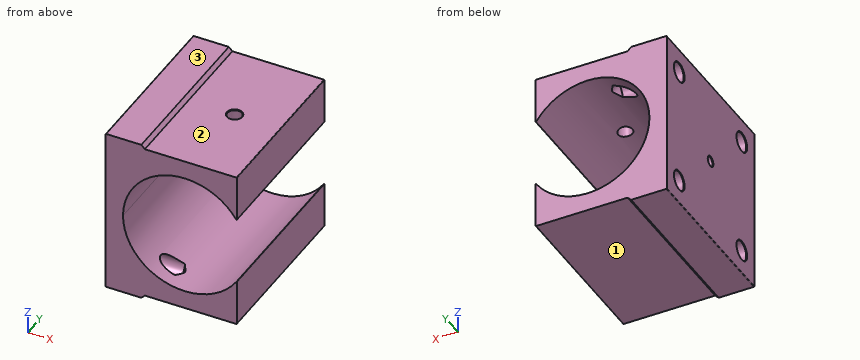
Autodesk Inventor part; units mm, degrees
ref_plane "YZ Plane" through (0, 0, 0) normal (1, 0, 0) x (0, 1, 0)
ref_plane "XZ Plane" through (0, 0, 0) normal (0, 1, 0) x (-1, 0, 0)
ref_plane "XY Plane" through (0, 0, 0) normal (0, 0, 1) x (1, 0, 0)
sketch "Boceto1" plane through (0, 0, 0) normal (0, 1, 0) x (-1, 0, 0)
  line L0 (10.2901, 15.6998) -> (10.2901, -54.8002)
  line L1 (10.2901, -54.8002) -> (-6.2099, -54.8002)
  line L2 (-44.9099, -53.3002) -> (-44.9099, 14.1998)
  line L3 (-6.2099, 15.6998) -> (10.2901, 15.6998)
  line L4 (10.2901, 15.6998) -> (-6.2099, 15.6998)
  line L5 (-6.2099, 15.6998) -> (-6.2099, 14.1998)
  line L6 (-6.2099, 14.1998) -> (-44.9099, 14.1998)
  line L7 (10.2901, -54.8002) -> (-6.2099, -54.8002)
  line L8 (-6.2099, -54.8002) -> (-6.2099, -53.3002)
  line L9 (-6.2099, -53.3002) -> (-44.9099, -53.3002)
  circle A0 centre (-23.0099, -19.5502) radius 26
  point P0 (0, 0)
  point P1 (-44.9099, -5.5363)
  point P2 (-44.9099, -33.5641)
  dimension "d0" = 70.5
  dimension "d3" = 16.5
  dimension "d4" = 1.5
  dimension "d5" = 1.5
  dimension "d6" = 55.2
  dimension "d7" = 67.5
  dimension "d8" = 52
  dimension "d9" = 33.3
  dimension "d10" = 33.75
extrude "Extrusión1" add sketch "Boceto1" along normal blind 70 contours L0 L1 L8 L9 L2 A0 L6 L5 L3
fillet "Empalme1" radius 0.25 2 edges at (-10.2901, 35, 15.6998) (-10.2901, 35, -54.8002)
chamfer "Chaflán1" distance 1.5 angle 45 1 edges at (6.2099, 35, 15.6998)
chamfer "Chaflán2" distance 1.5 angle 45 1 edges at (6.2099, 35, -54.8002)
sketch "Boceto2" plane through (-10.2901, 0, -54.5502) normal (-1, 0, 0) x (0, 0, 1)
  line L0 (9, 70) -> (61, 70)
  line L1 (35, 70) -> (35, 0)
  line L2 (0, 0) -> (70, 0)
  line L3 (35, 35) -> (-0.338, 35)
  line L4 (-0.338, 35) -> (70.438, 35)
  line L5 (35, 35) -> (59.975, 35)
  line L6 (35, 35) -> (10, 35)
  line L7 (10, 35) -> (10, 60)
  line L8 (10, 60) -> (60, 60)
  line L9 (60, 60) -> (60, 10)
  line L10 (60, 10) -> (10, 10)
  line L11 (10, 10) -> (10, 60)
  circle A0 centre (10, 60) radius 4
  circle A1 centre (60, 60) radius 4
  circle A2 centre (10, 10) radius 4
  circle A3 centre (60, 10) radius 4
  circle A4 centre (35, 35) radius 2
  point P0 (54.5502, 0)
  point P1 (49.0139, 70)
  point P2 (20.9861, 70)
  dimension "d23" = 25
  dimension "d24" = 50
  dimension "d25" = 50
  dimension "d26" = 8
  dimension "d27" = 8
  dimension "d28" = 8
  dimension "d29" = 8
  dimension "d30" = 4
  dimension "d73" = 25
hole "Agujero1" at (-10.2901, 60, -44.5502) at (-10.2901, 60, 5.4498) at (-10.2901, 10, -44.5502) at (-10.2901, 10, 5.4498) direction (1, 0, 0) diameter 8 depth 26 tip angle 118
thread "Rosca1"
thread "Rosca2"
thread "Rosca3"
thread "Rosca4"
hole "Agujero2" at (-10.2901, 35, -19.5502) direction (1, 0, 0) diameter 4 depth 26 tip angle 118
thread "Rosca5"
chamfer "Chaflán3" distance 0.25 angle 45 5 edges at (-10.2901, 60, -48.5502) (-10.2901, 60, 1.4498) (-10.2901, 10, -48.5502) (-10.2901, 10, 1.4498) (-10.2901, 35, -21.5502)
sketch "Boceto3" plane through (44.9099, 0, 14.1998) normal (0, 0, 1) x (1, 0, 0)
  point P0 (-44.9099, 0)
sketch "Boceto4" plane through (44.9099, 0, 14.1998) normal (0, 0, 1) x (1, 0, 0)
  line L0 (-38.7, 0) -> (-38.7, 70)
  line L1 (-38.7, 0) -> (-38.7, 70)
  line L2 (-47.9, 70) -> (0, 70)
  line L3 (-38.7, 70) -> (0, 70)
  line L4 (0, 0) -> (0, 70)
  line L5 (0, 70) -> (0, 0)
  line L6 (0, 0) -> (-38.7, 0)
  line L7 (-47.9, 0) -> (0, 0)
  line L8 (-19.35, 0) -> (-19.35, 70)
  line L9 (-19.35, 35) -> (-14.4981, 35)
  line L10 (-14.4981, 35) -> (-25.37, 35)
  circle A0 centre (-19.35, 35) radius 3
  point P0 (-44.9099, 0)
  dimension "d58" = 6
hole "Agujero3" at (25.5599, 35, 14.1998) direction (0, 0, -1) diameter 6 depth 26 tip angle 118
thread "Rosca6"
chamfer "Chaflán4" distance 0.25 angle 45 1 edges at (25.5599, 38, 14.1998)
fillet "Empalme2" radius 0.1 2 edges at (44.9099, 35, -5.5363) (44.9099, 35, -33.5641)
fillet "Empalme3" radius 0.2 2 edges at (44.9099, 35, -53.3002) (44.9099, 35, 14.1998)
properties part number "Soporte de Motor" material "Aluminio 6061"
Here's how the part is built. I have some questions about the finished solid (model axes, mm). Face numbers are marked on the shaded views. A direction names the side the tool comes from. Coordinates: 2 decimals unless noted, no trailing zeros. Write each loop counter-clockwise with the first axis right and the second up, starting at its lowest first coordinate (ties: lowest second). Pieces come first, ordered by that corner, then holes.
Item 1: Will these pins go through, and if not, where does the flat tip stop? pin 1 (6.5 mm diameter, centred on y = 60, z = 5.45, fed in from -X); pin 2 (5 mm diameter, centred on y = 10, z = -44.55, fed in from -X); pin 3 (10 mm diameter, centred on x = 34.5, y = 43, fed in from +Z); pin 4 (3.5 mm diameter, centred on y = 35, z = -19.55, fed in from +X).
Item 2: I want a section at D-D on z = -3. Write out the boundary of the cut face in (x, y).
Item 3: I want a section at B-B on x = -5. Write out the boundary of the cut face in (y, z), and give its area (3 significant figures).
Item 4: If I drill on line 1 (Z direction, x = -5.5, y = 35); line 2 (X direction, y = 35, z = 10.75); line 3 (Y direction, x = 1.5, z = 3), over which ranges is the centre line in solid material (lowest first)?
Item 5: On a 3-axis mill with a long thin cutter (end or side, diameter ignored), from which of +Z, -Z, +X, -X, +Y, -Y can I reach the whole of each face in a straight line? I mean the marked faces 1, 2 and 3. Say none if no direction works.
Item 6: I want a section at A-A on y = 60. Count the separate pieces of the cut face and the enclosed holes in it, and give its area (3 significant figures).
Item 7: I want a section at C-C on x = 35. Write out the boundary of the cut face in (y, z), and give its area (3 significant figures).
Findings below:
1. pin 1: stops at x = 16.16
1. pin 2: stops at x = 16.61
1. pin 3: stops at z = 14.2
1. pin 4: passes through
2. outline: (-10.29, 0) - (2.96, 0) - (2.96, 70) - (-10.29, 70) - close; (43.06, 0) - (44.91, 0) - (44.91, 70) - (43.06, 70) - close
3. outline: (0, -54.8) - (70, -54.8) - (70, 15.7) - (0, 15.7) - close; hole circle Ø8 at (10, -44.55); hole circle Ø8 at (10, 5.45); hole circle Ø4 at (35, -19.55); hole circle Ø8 at (60, -44.55); hole circle Ø8 at (60, 5.45)
3. area: 4,720 mm2
4. line 1: z = -54.8 to -21.55, -17.55 to 15.7
4. line 2: x = -10.29 to 22.56, 28.56 to 44.91
4. line 3: y = 0 to 6.84, 13.16 to 56.84, 63.16 to 70
5. face 1: -Z, +X, +Y, -Y
5. face 2: +Z, +X, +Y, -Y
5. face 3: +Z, +X, -X, +Y, -Y
6. separate pieces: 3
6. enclosed holes: 0
6. area: 1,340 mm2
7. outline: (0, -53.3) - (70, -53.3) - (70, -42.62) - (0, -42.62) - close; (0, 3.52) - (70, 3.52) - (70, 14.2) - (0, 14.2) - close
7. area: 1,500 mm2
